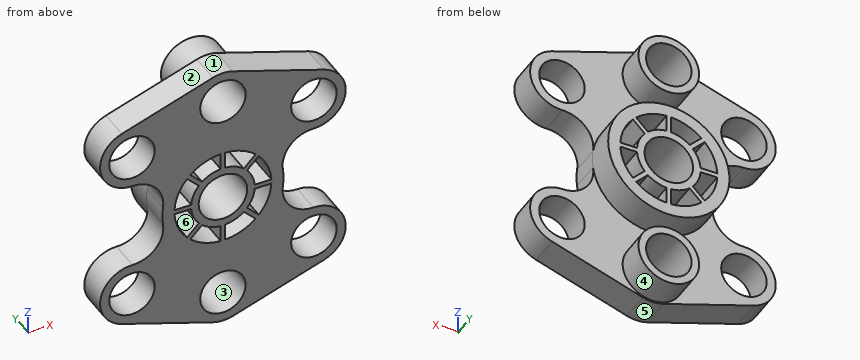
from build123d import *

# Parameters (mm, degrees)
BOSS_EXTRUDE2_DEPTH = 20
SKETCH2_R           = 40
SKETCH2_R_2         = 20
BOSS_EXTRUDE3_DEPTH = 20
SKETCH2_5_R         = 15
CUT_EXTRUDE1_DEPTH  = 20
SKETCH3_R           = 16
CUT_EXTRUDE2_DEPTH  = 129.226362344
SKETCH4_R           = 15
CUT_EXTRUDE3_DEPTH  = 129.226362344


with BuildPart() as part:
    # Sketch1 → Boss-Extrude2 (new body)
    with BuildSketch(Plane(origin=(0, 0, 0), x_dir=(1, 0, 0), z_dir=(0, 1, 0))):
        with BuildLine():
            Line((-66.640783086, 69.922349259), (-6.640783086, 89.922349259))
            ThreePointArc((-6.640783086, 89.922349259), (0, 91), (6.640783086, 89.922349259))
            Line((6.640783086, 89.922349259), (66.640783086, 69.922349259))
            ThreePointArc((66.640783086, 69.922349259), (80.700240831, 46.464461919), (59.651863383, 29.002885891))
            ThreePointArc((59.651863383, 29.002885891), (44.262528341, 22.168588856), (39.546869801, 6.003756239))
            ThreePointArc((39.546869801, 6.003756239), (40, 0), (39.546869801, -6.003756239))
            ThreePointArc((39.546869801, -6.003756239), (44.262528341, -22.168588856), (59.651863383, -29.002885891))
            ThreePointArc((59.651863383, -29.002885891), (80.700240831, -46.464461919), (66.640783086, -69.922349259))
            Line((66.640783086, -69.922349259), (6.640783086, -89.922349259))
            ThreePointArc((6.640783086, -89.922349259), (0, -91), (-6.640783086, -89.922349259))
            Line((-6.640783086, -89.922349259), (-66.640783086, -69.922349259))
            ThreePointArc((-66.640783086, -69.922349259), (-80.700240831, -46.464461919), (-59.651863383, -29.002885891))
            ThreePointArc((-59.651863383, -29.002885891), (-44.262528341, -22.168588856), (-39.546869801, -6.003756239))
            ThreePointArc((-39.546869801, -6.003756239), (-40, 0), (-39.546869801, 6.003756239))
            ThreePointArc((-39.546869801, 6.003756239), (-44.262528341, 22.168588856), (-59.651863383, 29.002885891))
            ThreePointArc((-59.651863383, 29.002885891), (-80.700240831, 46.464461919), (-66.640783086, 69.922349259))
        make_face()
    extrude(amount=BOSS_EXTRUDE2_DEPTH)

    # Sketch2 → Boss-Extrude3 (add)
    with BuildSketch(Plane(origin=(0, 20, 0), x_dir=(1, 0, 0), z_dir=(0, 1, 0))):
        with Locations(Location((0, 0, 0), (0, 0, 8.632368585))):
            Circle(SKETCH2_R)
        with Locations(Location((0, 70, 0), (0, 0, 90))):
            Circle(SKETCH2_R_2)
        with Locations(Location((0, -70, 0), (0, 0, 270))):
            Circle(SKETCH2_R_2)
    extrude(amount=BOSS_EXTRUDE3_DEPTH)

    # Sketch2_5 → Cut-Extrude1 (cut)
    with BuildSketch(Plane(origin=(0, 20, 0), x_dir=(1, 0, 0), z_dir=(0, 1, 0))):
        with Locations(Location((60, 50, 0), (0, 0, 270))):
            Circle(SKETCH2_5_R)
        with Locations(Location((-60, 50, 0), (0, 0, 270))):
            Circle(SKETCH2_5_R)
        with Locations(Location((60, -50, 0), (0, 0, 270))):
            Circle(SKETCH2_5_R)
        with Locations(Location((-60, -50, 0), (0, 0, 270))):
            Circle(SKETCH2_5_R)
    extrude(amount=-CUT_EXTRUDE1_DEPTH, mode=Mode.SUBTRACT)

    # Sketch3 → Cut-Extrude2 (cut, through all)
    with BuildSketch(Plane(origin=(0, 40, 0), x_dir=(1, 0, 0), z_dir=(0, 1, 0))):
        with Locations(Location((0, 0, 0), (0, 0, 270))):
            Circle(SKETCH3_R)
        with BuildLine():
            Line((-1.5, 31.964824417), (-1.5, 20.946360066))
            ThreePointArc((-1.5, 20.946360066), (-8.03635208, 19.401470183), (-13.750653072, 15.871973415))
            Line((-13.750653072, 15.871973415), (-21.541883933, 23.663204276))
            ThreePointArc((-21.541883933, 23.663204276), (-12.245869836, 29.56414504), (-1.5, 31.964824417))
        make_face()
        with BuildLine():
            Line((1.5, 31.964824417), (1.5, 20.946360066))
            ThreePointArc((1.5, 20.946360066), (8.03635208, 19.401470183), (13.750653072, 15.871973415))
            Line((13.750653072, 15.871973415), (21.541883933, 23.663204276))
            ThreePointArc((21.541883933, 23.663204276), (12.245869836, 29.56414504), (1.5, 31.964824417))
        make_face()
        with BuildLine():
            Line((23.663204276, 21.541883933), (15.871973415, 13.750653072))
            ThreePointArc((15.871973415, 13.750653072), (19.401470183, 8.03635208), (20.946360066, 1.5))
            Line((20.946360066, 1.5), (31.964824417, 1.5))
            ThreePointArc((31.964824417, 1.5), (29.56414504, 12.245869836), (23.663204276, 21.541883933))
        make_face()
        with BuildLine():
            Line((31.964824417, -1.5), (20.946360066, -1.5))
            ThreePointArc((20.946360066, -1.5), (19.401470183, -8.03635208), (15.871973415, -13.750653072))
            Line((15.871973415, -13.750653072), (23.663204276, -21.541883933))
            ThreePointArc((23.663204276, -21.541883933), (29.56414504, -12.245869836), (31.964824417, -1.5))
        make_face()
        with BuildLine():
            Line((21.541883933, -23.663204276), (13.750653072, -15.871973415))
            ThreePointArc((13.750653072, -15.871973415), (8.03635208, -19.401470183), (1.5, -20.946360066))
            Line((1.5, -20.946360066), (1.5, -31.964824417))
            ThreePointArc((1.5, -31.964824417), (12.245869836, -29.56414504), (21.541883933, -23.663204276))
        make_face()
        with BuildLine():
            Line((-1.5, -31.964824417), (-1.5, -20.946360066))
            ThreePointArc((-1.5, -20.946360066), (-8.03635208, -19.401470183), (-13.750653072, -15.871973415))
            Line((-13.750653072, -15.871973415), (-21.541883933, -23.663204276))
            ThreePointArc((-21.541883933, -23.663204276), (-12.245869836, -29.56414504), (-1.5, -31.964824417))
        make_face()
        with BuildLine():
            Line((-23.663204276, -21.541883933), (-15.871973415, -13.750653072))
            ThreePointArc((-15.871973415, -13.750653072), (-19.401470183, -8.03635208), (-20.946360066, -1.5))
            Line((-20.946360066, -1.5), (-31.964824417, -1.5))
            ThreePointArc((-31.964824417, -1.5), (-29.56414504, -12.245869836), (-23.663204276, -21.541883933))
        make_face()
        with BuildLine():
            Line((-31.964824417, 1.5), (-20.946360066, 1.5))
            ThreePointArc((-20.946360066, 1.5), (-19.401470183, 8.03635208), (-15.871973415, 13.750653072))
            Line((-15.871973415, 13.750653072), (-23.663204276, 21.541883933))
            ThreePointArc((-23.663204276, 21.541883933), (-29.56414504, 12.245869836), (-31.964824417, 1.5))
        make_face()
    extrude(amount=-CUT_EXTRUDE2_DEPTH, mode=Mode.SUBTRACT)

    # Sketch4 → Cut-Extrude3 (cut, through all)
    with BuildSketch(Plane(origin=(0, 40, 0), x_dir=(1, 0, 0), z_dir=(0, 1, 0))):
        with Locations(Location((0, 70, 0), (0, 0, 270))):
            Circle(SKETCH4_R)
        with Locations(Location((0, -70, 0), (0, 0, 270))):
            Circle(SKETCH4_R)
    extrude(amount=-CUT_EXTRUDE3_DEPTH, mode=Mode.SUBTRACT)


solid = part.part
CAD build for the part. Positions are in the model's coordinates, mm. Face numbers are marked on the shaded views. A direction names the side the tool comes from. Coordinates: 2 decimals unless noted, no trailing zeros. Write each loop counter-clockwise with the first axis right and the second up, starting at its lowest first coordinate (ties: lowest second). Pieces come first, ordered by that corner, then holes. Notation, with made-up numbers: (-29.5, 82) - (-7.5, 82) arc R19 ccw to (-7.5, 99) - close; hole circle Ø8 at (26.5, 76). An arc over 180 degrees is marked (long way). Use a Markdown table: item, result. Add a question column.
Item 1: Band-saw the part on A-A, the plane z = 10.5. Give the cut face in (x, y).
Item 2: Band-saw the part on D-D, the plane z = 44. Give the cut face in (x, y).
Item 3: 3-axis set-ups, long thin cutter, end or side, ignore diameter. For the marked faces 4, 5 and 6: which of +Z, -Z, +X, -X, +Y, -Y reach the whole face in a straight line?
Item 4: Drill centre lines: L1, parallel to X at y = 22, z = 6.5; L2, parallel to X at y = 7, z = 50; L3, parallel to X at y = 5, z = 18. Where is each one in solid material? Low to high. Write a range as from..to.
Item 5: Mould opens along X. For the marked faces 1, 2 and 3 say: pulls with the +X half, pulls with the -X half, needs draft (parallel to the pull), parting line crosses it, or undercut.
Item 6: Band-saw the part on B-B, the plane x = -62.5. Give the cut face in (y, z).
Item 7: Band-saw the part on C-C, the plane y = 33. Give the number of separate pieces and of enclosed holes in the cut face, and give its area (3 significant figures).
Item 8: Flat gauge pins, fed straight in: pin 1 (1 mm diameter, centred on x = 32.5, y = 21.5, fed in from -Z); pin 2 (12 mm diameter, centred on y = 27, z = -24.5, fed in from -X); pin 3 (4 mm diameter, centred on x = -44.5, y = 17, fed in from +Z). Where does each tip first touch, or does it go through?
Numbers:
| question | item | result |
|---|---|---|
| 1 | outline | (-39.38, 0) - (-30.23, 0) - (-30.23, 40) - (-38.6, 40) - (-38.6, 20) - (-39.38, 20) - close; (-18.19, 0) - (-12.07, 0) - (-12.07, 40) - (-18.19, 40) - close; (12.07, 0) - (18.19, 0) - (18.19, 40) - (12.07, 40) - close; (30.23, 0) - (39.38, 0) - (39.38, 20) - (38.6, 20) - (38.6, 40) - (30.23, 40) - close |
| 2 | outline | (-80.12, 0) - (-73.75, 0) - (-73.75, 20) - (-80.12, 20) - close; (-46.25, 0) - (46.25, 0) - (46.25, 20) - (-46.25, 20) - close; (73.75, 0) - (80.12, 0) - (80.12, 20) - (73.75, 20) - close |
| 3 | face 4 | +Y |
| 3 | face 5 | -Z, +Y, -Y |
| 3 | face 6 | +Y, -Y |
| 4 | L1 | -39.47..-31.33, -19.97..-14.62, 14.62..19.97, 31.33..39.47 |
| 4 | L2 | -81..-75, -45..45, 75..81 |
| 4 | L3 | -41.46..-26.46, -20.12..-15.88, -10.82..10.82, 15.88..20.12, 26.46..41.46 |
| 5 | face 1 | parting line crosses it |
| 5 | face 2 | pulls with the -X half |
| 5 | face 3 | undercut |
| 6 | outline | (0, -71.3) - (20, -71.3) - (20, -64.79) - (0, -64.79) - close; (0, -35.21) - (20, -35.21) - (20, -29.15) - (0, -29.15) - close; (0, 29.15) - (20, 29.15) - (20, 35.21) - (0, 35.21) - close; (0, 64.79) - (20, 64.79) - (20, 71.3) - (0, 71.3) - close |
| 7 | separate pieces | 3 |
| 7 | enclosed holes | 11 |
| 7 | area | 3,750 mm2 |
| 8 | pin 1 | z = -24 |
| 8 | pin 2 | x = -35.46 |
| 8 | pin 3 | z = 77.97 |
